```python
from build123d import *

# Parameters (mm, degrees)
SKETCH1_R      = 25.527
SKETCH1_R_2    = 2.5781
EXTRUDE1_DEPTH = 4.7752


with BuildPart() as part:
    # Sketch1 → Extrude1 (new body)
    with BuildSketch(Plane.XY):
        with BuildLine():
            Line((-28.575, 38.1), (28.575, 38.1))
            ThreePointArc((28.575, 38.1), (35.310192091, 35.310192091), (38.1, 28.575))
            Line((38.1, 28.575), (38.1, -28.575))
            ThreePointArc((38.1, -28.575), (35.310192091, -35.310192091), (28.575, -38.1))
            Line((28.575, -38.1), (-28.575, -38.1))
            ThreePointArc((-28.575, -38.1), (-35.310192091, -35.310192091), (-38.1, -28.575))
            Line((-38.1, -28.575), (-38.1, 28.575))
            ThreePointArc((-38.1, 28.575), (-35.310192091, 35.310192091), (-28.575, 38.1))
        make_face()
        Circle(SKETCH1_R, mode=Mode.SUBTRACT)
        with Locations((-28.575, 28.575)):
            Circle(SKETCH1_R_2, mode=Mode.SUBTRACT)
        with Locations(Location((28.575, 28.575, 0), (0, 0, 180))):
            Circle(SKETCH1_R_2, mode=Mode.SUBTRACT)
        with Locations(Location((-28.575, -28.575, 0), (0, 0, 180))):
            Circle(SKETCH1_R_2, mode=Mode.SUBTRACT)
        with Locations((28.575, -28.575)):
            Circle(SKETCH1_R_2, mode=Mode.SUBTRACT)
    extrude(amount=-EXTRUDE1_DEPTH)


solid = part.part
```
Geometry check sheet. Reference: the model listing, model coordinates, mm. Coordinates: 2 decimals unless noted, no trailing zeros. Write each loop counter-clockwise with the first axis right and the second up, starting at its lowest first coordinate (ties: lowest second). Pieces come first, ordered by that corner, then holes. Notation, with made-up numbers: (66.5, 62.5) -> (105.5, 62.5) arc R27 cw to (105.5, 91.5) -> close; hole circle Ø11 at (18, 4). An arc over 180 degrees is marked (long way). Use CSV: the item, a comma, the result in double quotes. Start each with the question number.
Item 1: Thickness scan on line 1 (Y direction, x = 27.5, z = -1.7); line 2 (Y direction, x = 0, z = -1.75); line 3 (Y direction, x = 9, z = -3.95). Record the ranges inside material, lowest first.
Item 2: Mould release check, pull along X, two halves, no side actions. Record for faces 1 (the flat face through (38.1, 0, -2)), 2 (the cylindrical face through (24.348, 7.668, -2.354)), 3 (the flat face through (1, 26, -4.775)): released by +X, released by -X, zero draft, split by the parting line, or undercut.
Item 3: Cross-section at D-D, the plane x = -29.5. Record the cut outline in (y, z).
Item 4: Cross-section at A-A, the plane y = 0. Record the cut outline in (x, z), plus the area to 3 significant figures.
Item 5: Cross-section at C-C, the plane z = -2.1. Record the cut outline in (x, y) (3 decimals).
Answers:
1,line 1,"-38.1 to -30.92, -26.23 to 26.23, 30.92 to 38.1"
1,line 2,"-38.1 to -25.53, 25.53 to 38.1"
1,line 3,"-38.1 to -23.89, 23.89 to 38.1"
2,face 1,"released by +X"
2,face 2,"undercut"
2,face 3,"zero draft"
3,outline,"(-38.05, -4.78) -> (-30.98, -4.78) -> (-30.98, 0) -> (-38.05, 0) -> close; (-26.17, -4.78) -> (26.17, -4.78) -> (26.17, 0) -> (-26.17, 0) -> close; (30.98, -4.78) -> (38.05, -4.78) -> (38.05, 0) -> (30.98, 0) -> close"
4,outline,"(-38.1, -4.78) -> (-25.53, -4.78) -> (-25.53, 0) -> (-38.1, 0) -> close; (25.53, -4.78) -> (38.1, -4.78) -> (38.1, 0) -> (25.53, 0) -> close"
4,area,"120 mm^2"
5,outline,"(-38.1, -28.575) arc R9.525 ccw to (-28.575, -38.1) -> (28.575, -38.1) arc R9.525 ccw to (38.1, -28.575) -> (38.1, 28.575) arc R9.525 ccw to (28.575, 38.1) -> (-28.575, 38.1) arc R9.525 ccw to (-38.1, 28.575) -> close; hole circle Ø5.156 at (-28.575, -28.575); hole circle Ø5.156 at (-28.575, 28.575); hole circle Ø51.054 at (0, 0); hole circle Ø5.156 at (28.575, -28.575); hole circle Ø5.156 at (28.575, 28.575)"
